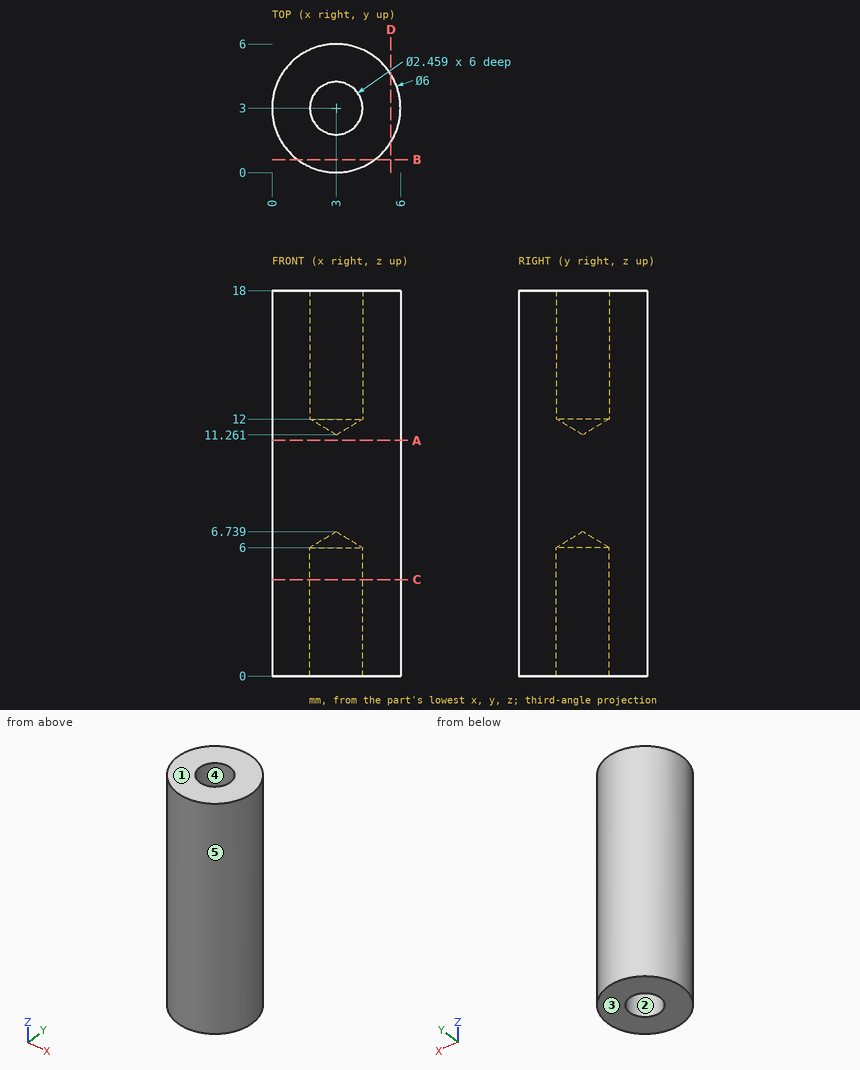
The figure shows three views and two pictorial views of one solid part (mm, origin at its lowest corner). Answer the questions. A direction names the side the tool comes from. Give positions to 0.01 mm unless a question says otherwise; leave off trailing zeros. Loops run counter-clockwise (first coordinate to the right, second up) from the corner with the lowest first, then second, coordinate; pieces in that order, holes last. Notation, with made-up numbers: M 79,44.5 L 112,44.5 A21 cw 112,80.5 Z; hole C -9,55 d5. An arc over 180 degrees is marked long. Write each question's results on one line, items separated by ' | '.
1. Section B-B on y = 0.6 is taken. Give the vertices of the cut face in (x, z), plus the area to 3 significant figures.
Values:
outline: M 1.2,0 L 4.8,0 L 4.8,18 L 1.2,18 Z | area: 64.8 mm^2
2. Section D-D on x = 5.55 is taken. Give the vertices of the cut face in (y, z), plus the area to 3 significant figures.
Values:
outline: M 1.42,0 L 4.58,0 L 4.58,18 L 1.42,18 Z | area: 56.9 mm^2
3. The mould has two halves that part along Y. Classify the marked faces 3, 4 and 5: pulls with the +Y half, pulls with the -Y half, needs draft (parallel to the pull), parting line crosses it, or undercut.
Values:
face 3: needs draft | face 4: undercut | face 5: parting line crosses it
4. Section C-C on z = 4.5 is taken. Give the vertices of the cut face in (x, y).
Values:
outline: C 3,3 d6; hole C 3,3 d2.46
5. Straight lines are drawn through the part: line 1 (Y direction, x = 3, z = 4.45); line 2 (Y direction, x = 2.85, z = 7.75); line 3 (X direction, y = 3.8, z = 15.5). For each, find the intervals that lie inside material, in ascending order. Write a range as [from, to].
Values:
line 1: y = [0, 1.77], [4.23, 6] | line 2: y = [0, 6] | line 3: x = [0.11, 2.07], [3.93, 5.89]
6. A tool of negligible diameter and unlimited length cuts with its end or side. For the marked faces 1 and 2, from which of +Z, -Z, +X, -X, +Y, -Y can it reach the whole face along a straight path? Write none if from no direction.
Values:
face 1: +Z, +X, -X, +Y, -Y | face 2: -Z
7. Section A-A on z = 11 is taken. Give the vertices of the cut face in (x, y), plus the area to 3 significant figures.
Values:
outline: C 3,3 d6 | area: 28.3 mm^2
8. Given pin 1 (1 mm diameter, centred on x = 5, z = 4, fed in from +Y); pin 2 (2 mm diameter, centred on x = 3, y = 3, fed in from +Z), each flat-ended and moving along its own axis, determine where each tip first touches the part or whether it passes through.
Values:
pin 1: stops at y = 5.6 | pin 2: stops at z = 11.86
